The listing builds one solid part. Answer for the finished solid, in the listing's coordinates (mm). Face numbers are marked on the shaded views. A direction names the side the tool comes from. Round coordinates to 2 decimals unless told otherwise and drop trailing zeros. Write each loop counter-clockwise with the first axis right and the second up, starting at its lowest first coordinate (ties: lowest second). Pieces come first, ordered by that corner, then holes.
(1) A cutting plane is placed at D-D, the plane z = 7. Give the vertices of the cut face in (x, y), and give its area (3 significant figures).
(2) The mould has two halves that part along X. Classify the marked faces 1, 2 and 3: +X half, -X half, draft (parallel to the pull), parting line (faces both ways), or undercut.
(3) A cutting plane is placed at B-B, the plane y = 6. Give the vertices of the cut face in (x, z).
(4) For the marked faces 4, 5 and 6, determine the directions among +Z, -Z, +X, -X, +Y, -Y from which every point of the face is accessible in a straight line to the end or side of a thin tool.
(5) Find the intervals of material crossed by probe 1 along Y at (x, z) = (0, -8); probe 2 along X at (y, z) = (2, -7.5); probe 3 along Z at (x, y) = (28.5, 8.5), in increasing order.
(6) Each of these flat-tipped pins is pushed along its axis until it touches: pin 1 Ø8 at (x, z) = (11, -1) entering from -Y; pin 2 Ø10 at (y, z) = (30, -2.5) entering from +X; pin 3 Ø6 at (x, z) = (-26.5, -7) entering from +Y; pin 4 Ø3 at (y, z) = (18, -11.5) entering from +X. Where does it stop, or does it pass through?
(7) A cutting plane is placed at C-C, the plane z = -13. Give the vertices of the cut face in (x, y), and give its area (3 significant figures).
(8) A cutting plane is placed at A-A, the plane x = 0. Give the vertices of the cut face in (y, z).
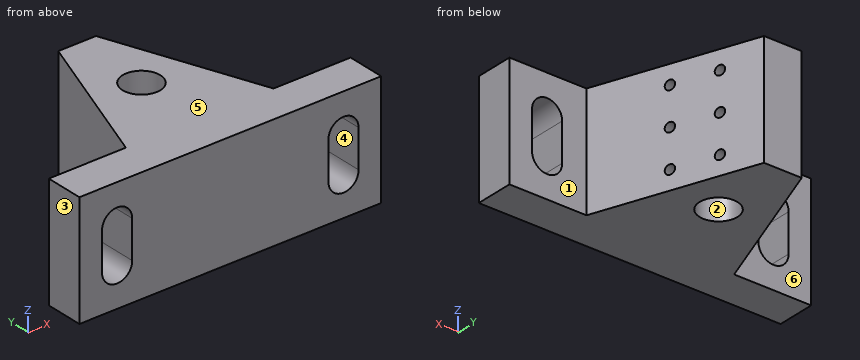
from build123d import *

# Parameters (mm, degrees)
BASE_EXTRUDE_DEPTH   = 15
SLOT_CUT_DEPTH       = 66.76473219
SKETCH5_R            = 5
GUIDE_HOLE_DEPTH     = 71.710678119
LPATTERN1_COUNT      = 3
LPATTERN1_PITCH      = 10
LPATTERN1_COUNT_DIR2 = 2
LPATTERN1_PITCH_DIR2 = 12


with BuildPart() as part:
    # Sketch2 → Base Extrude (new, symmetric)
    with BuildSketch(Plane.XY):
        Polygon((-40, 0), (40, 0), (40, 10), (19.558809371, 10), (5, 50), (-5, 50), (-19.558809371, 10), (-40, 10), align=None)
    extrude(amount=BASE_EXTRUDE_DEPTH, both=True)

    # Sketch4 → Slot Cut (cut, through all)
    with BuildSketch(Plane(origin=(0, 0, 0), x_dir=(1, 0, 0), z_dir=(0, 1, 0))):
        with BuildLine():
            Line((26, -5), (26, 5))
            ThreePointArc((26, 5), (30, 9), (34, 5))
            Line((34, 5), (34, -5))
            ThreePointArc((34, -5), (30, -9), (26, -5))
        make_face()
    slot_cut = extrude(amount=SLOT_CUT_DEPTH, mode=Mode.SUBTRACT)

    # Mirror1: Slot Cut across plane
    add(slot_cut.mirror(Plane(origin=(0, 0, 0), x_dir=(0, 0, 1), z_dir=(1, 0, 0))), mode=Mode.SUBTRACT)

    # Sketch5 → Guide Hole (cut, through all)
    with BuildSketch(Plane.XY.offset(15)):
        with Locations((0, 29)):
            Circle(SKETCH5_R)
    extrude(amount=-GUIDE_HOLE_DEPTH, mode=Mode.SUBTRACT)

    # Sketch10 → M3x0.5 Tapped Hole2 (revolve, cut)
    with BuildSketch(Plane(origin=(12.718406504, 28.793852416, 10), x_dir=(-0.3420201433256662, 0.9396926207859093, 0), z_dir=(0, 0, 1))):
        Polygon((0, 0), (0, 8.251075774), (1.25, 7.5), (1.25, 0), align=None)
    m3x0_5_tapped_hole2 = revolve(axis=Axis((18.685454646, 30.965680326, 10), (-0.9396926207859093, -0.34202014332566616, 0)), mode=Mode.SUBTRACT)

    # LPattern1: M3x0.5 Tapped Hole2 3 × 2
    with Locations(*[Vector(0, 0, -1) * (i * LPATTERN1_PITCH) + Vector(-0.34202014332566616, 0.9396926207859094, 0) * (j * LPATTERN1_PITCH_DIR2) for i in range(LPATTERN1_COUNT) for j in range(LPATTERN1_COUNT_DIR2) if (i, j) != (0, 0)]):
        add(m3x0_5_tapped_hole2, mode=Mode.SUBTRACT)


solid = part.part
Solutions:
1. outline: (-40, 0) - (-33.46, 0) - (-33.46, 10) - (-40, 10) - close; (-26.54, 0) - (26.54, 0) - (26.54, 10) - (19.56, 10) - (5, 50) - (-5, 50) - (-19.56, 10) - (-26.54, 10) - close; (33.46, 0) - (40, 0) - (40, 10) - (33.46, 10) - close; hole circle Ø10 at (0, 29)
1. area: 1,570 mm2
2. face 1: draft
2. face 2: undercut
2. face 3: -X half
3. outline: (-40, -15) - (40, -15) - (40, 15) - (-40, 15) - close; hole (-34, -5) arc R4 ccw to (-26, -5) - (-26, 5) arc R4 ccw to (-34, 5) - close; hole (26, -5) arc R4 ccw to (34, -5) - (34, 5) arc R4 ccw to (26, 5) - close
4. face 4: +Y, -Y
4. face 5: +Z, +X, -X, +Y, -Y
4. face 6: +Z, -Z, -X, +Y
5. probe 1: y = 0 to 24, 34 to 50
5. probe 2: x = -40 to -33.12, -26.88 to 26.88, 33.12 to 40
5. probe 3: z = -15 to -8.71, 8.71 to 15
6. pin 1: stops at y = 0
6. pin 2: stops at x = 14.1
6. pin 3: stops at y = 10
6. pin 4: stops at x = 17.19
7. outline: (-40, 0) - (40, 0) - (40, 10) - (19.56, 10) - (5, 50) - (-5, 50) - (-19.56, 10) - (-40, 10) - close; hole circle Ø10 at (0, 29)
7. area: 1,700 mm2
8. outline: (0, -15) - (24, -15) - (24, 15) - (0, 15) - close; (34, -15) - (50, -15) - (50, 15) - (34, 15) - close
